Here's how the part is built. I have some questions about the finished solid (model axes, mm). A direction names the side the tool comes from. Give positions to 0.01 mm unless a question says otherwise; leave off trailing zeros. Order: outer loops, then holes, each group sorted by start corner. A loop starts at its lowest first (then second) coordinate and runs counter-clockwise, first axis right, second up. Notation, with made-up numbers: (42.5, 71.25) -> (76.5, 71.25) arc R16 cw to (76.5, 77.25) -> close; hole circle Ø11 at (5, -30). An arc over 180 degrees is marked (long way). Write each question's results on one line, items separated by ' | '. Start each with the question number.
Q1. Imagine slicing it at D-D, the plane y = 32.5. Please give me the cut outline in (x, z), then the cut area to 3 significant figures.
Q2. For faces 5 (the face through (-5.067, 38.525, 95.719)), 6 (the face through (17, -17, 0)), which set-ups out of +Z, -Z, +X, -X, +Y, -Y let a thin tool reach every point of the face, with its end or its side?
Q3. Imagine slicing it at B-B, the plane x = 0. Please give me the cut outline in (y, z).
Q4. Imagine slicing it at A-A, the plane y = 0. Please give me the cut outline in (x, z), then the cut area to 3 significant figures.
Q5. Thinking about a two-plate mould opening in X: for faces 1 (the face through (-16.597, 32.655, 78.126)), 2 (the face through (11.65, 40.91, 95.3)), 3 (the face through (-5.149, 23.185, 71.879)), 4 (the face through (17, -17, 145.8)), which applies, pulls with the +X half, pulls with the -X half, needs draft (parallel to the pull), parting line crosses it, or undercut?
Q6. I need wall thicknesses on line 1 along Z through (x, y) = (-1, 28); line 2 along X through (y, z) = (33, 72.9); line 3 along Y through (x, z) = (6.5, 122.5). Which ranges of each line are inside material? Lowest first, please. Write a range as [from, to].
Q7. I'm going to push flat-ended pins straight in: pin 1 (6 mm diameter, centred on y = 16.5, z = 109.5, fed in from +X); pin 2 (8 mm diameter, centred on x = -15.5, y = 7.5, fed in from -Z); pin 3 (1.5 mm diameter, centred on y = -18, z = 82.5, fed in from -X); pin 4 (1.5 mm diameter, centred on y = -15.5, z = 31, fed in from -X). Where does each tip first touch, or does it pass through?
Q8. Imagine slicing it at C-C, the plane z = 115.5. Please give me the cut outline in (x, y), then the cut area to 3 significant figures.
Autodesk Inventor part; units mm, degrees
ref_plane "Work Plane1" through (0, 41.4, 0) normal (0, 1, 0) x (-1, 0, 0)
ref_plane "YZ Plane" through (0, 0, 0) normal (1, 0, 0) x (0, 1, 0)
ref_plane "XZ Plane" through (0, 0, 0) normal (0, 1, 0) x (-1, 0, 0)
sketch "Sketch1" plane through (0, 0, 0) normal (0, 0, 1) x (1, 0, 0)
  circle A0 centre (0, 0) radius 25.4
  circle A1 centre (0, 0) radius 23.75
  dimension "d0" = 50.8
  dimension "d1" = 1.65
extrude "Extrusion1" add sketch "Sketch1" along normal blind 145.8
ref_plane "Work Plane1" through (0, 41.4, 0) normal (0, 1, 0) x (-1, 0, 0)
sketch "Sketch2" plane through (0, 41.4, 0) normal (0, 1, 0) x (-1, 0, 0)
  line L0 (-25.4, 145.8) -> (25.4, 145.8)
  line L1 (-25.4, 145.8) -> (25.4, 145.8)
  line L2 (-25.4, 0) -> (25.4, 0)
  line L3 (25.4, 0) -> (25.4, 145.8)
  line L4 (-25.4, 0) -> (-25.4, 145.8)
  line L5 (0, 145.8) -> (0, 0) construction
  circle A0 centre (0, 72.9) radius 19.05
  circle A1 centre (0, 72.9) radius 17.4
  dimension "d5" = 38.1
  dimension "d7" = 1.65
extrude "Extrusion2" add sketch "Sketch2" against normal up to next contours A0
sketch "Sketch3" plane through (0, 41.4, 72.9) normal (0, 1, 0) x (1, 0, 0)
  circle A0 centre (0, 0) radius 19.05
  circle A1 centre (0, 0) radius 25.25
  dimension "d10" = 50.5
extrude "Extrusion3" add sketch "Sketch3" against normal blind 3
chamfer "Chamfer1" distance 2 angle 45 1 edges at (-25.25, 38.4, 72.9)
properties part number "ASME BPE Red Inst Tee-50.8-38.1"
Geometry check:
1) outline: circle Ø38.1 at (0, 72.9); hole circle Ø34.8 at (0, 72.9) | area: 189 mm²
2) face 5: none | face 6: -Z, +X, -X, +Y, -Y
3) outline: (-25.4, 0) -> (-23.75, 0) -> (-23.75, 145.8) -> (-25.4, 145.8) -> close; (23.75, 0) -> (25.4, 0) -> (25.4, 53.85) -> (38.4, 53.85) -> (38.4, 49.65) -> (40.4, 47.65) -> (41.4, 47.65) -> (41.4, 55.5) -> (25.4, 55.5) -> (25.4, 90.3) -> (41.4, 90.3) -> (41.4, 98.15) -> (40.4, 98.15) -> (38.4, 96.15) -> (38.4, 91.95) -> (25.4, 91.95) -> (25.4, 145.8) -> (23.75, 145.8) -> close
4) outline: (-25.4, 0) -> (-23.75, 0) -> (-23.75, 145.8) -> (-25.4, 145.8) -> close; (23.75, 0) -> (25.4, 0) -> (25.4, 145.8) -> (23.75, 145.8) -> close | area: 481 mm²
5) face 1: undercut | face 2: parting line crosses it | face 3: undercut | face 4: needs draft
6) line 1: [53.88, 55.53], [90.27, 91.92] | line 2: [-19.05, -17.4], [17.4, 19.05] | line 3: [-24.55, -22.84], [22.84, 24.55]
7) pin 1: x = 21.52 | pin 2: through | pin 3: x = -18.64 | pin 4: x = -20.68
8) outline: circle Ø50.8 at (0, 0); hole circle Ø47.5 at (0, 0) | area: 255 mm²
